```python
from build123d import *

# Parameters (mm, degrees)
F0_W     = 76.2
F0_H     = 177.8
F1_DEPTH = 12.7
F3_D     = 7.62
F4_D     = 7.62
F6_W     = 53.435474
F6_H     = 112.436191
F6_R     = 15.902152
F7_DEPTH = 36.66461


with BuildPart() as f1:
    # F0 (on Top) → F1 (new body)
    with BuildSketch(Plane.XY):
        with Locations((-11.308188, 0.622381)):
            Rectangle(F0_W, F0_H)
    extrude(amount=F1_DEPTH)

    # F3 (through all)
    with Locations(Plane.YZ.offset(26.791812)):
        with Locations((-79.060733, 6.35)):
            Hole(F3_D / 2)

    # F4 (through all)
    with Locations(Plane.YZ.offset(26.791812)):
        with Locations((80.305494, 6.35)):
            Hole(F4_D / 2)

    # F6 (on face) → F7 (join)
    with BuildSketch(Plane.XY.offset(12.7)):
        with Locations((-13.522789, 21.443374)):
            Rectangle(F6_W, F6_H)
        with Locations((-13.522789, 21.443374)):
            Circle(F6_R, mode=Mode.SUBTRACT)
    extrude(amount=F7_DEPTH)


solid = f1.part
```
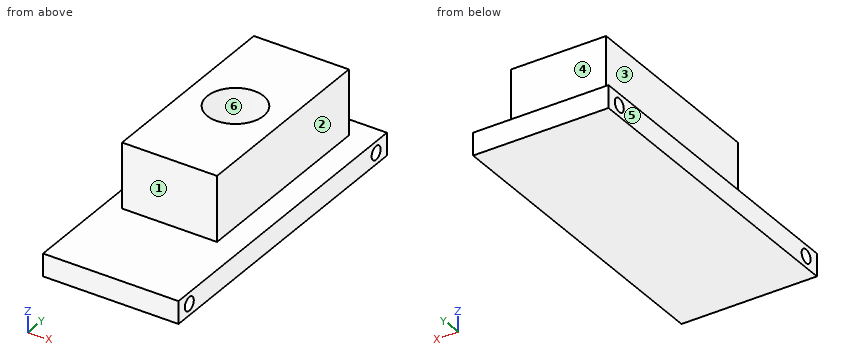
Work out the finished part from the listing and answer in its coordinate system (mm). Face numbers are marked on the shaded views. A direction names the side the tool comes from. Give positions to 0.01 mm unless a question says otherwise; leave off trailing zeros. Loops run counter-clockwise (first coordinate to the right, second up) from the corner with the lowest first, then second, coordinate; pieces in that order, holes last. Notation, with made-up numbers: (17.5, 45) -> (56.5, 45) arc R25 cw to (56.5, 78) -> close; hole circle Ø10 at (-26.5, 36). An arc over 180 degrees is marked (long way). Put each result on its own line as item: value. Start each with the question number.
Item 1: Find the intervals of material crossed by L1, parallel to Y at x = -17, z = 6; L2, parallel to Y at x = -42, z = 3; L3, parallel to Z at x = -29, y = -65, in increasing order. Write a range as [from, to].
Item 2: The mould has two halves that part along Y. Classify the marked faces 4, 5 and 6: released by +Y, released by -Y, zero draft, split by the parting line, or undercut.
Item 3: The part is cut by section B-B (x = -38). Give the vertices of the cut face in (y, z), then the cut area to 3 significant figures.
Item 4: The part is cut by section A-A (z = 6.35). Give the vertices of the cut face in (x, y).
Item 5: The part is cut by section D-D (x = 21.5). Give the vertices of the cut face in (y, z), then the cut area to 3 significant figures.
Item 6: Which of the six approach directions +Z, -Z, +X, -X, +Y, -Y give full straight-line access (tool end or side, diameter ignored) to the marked faces 1, 2 and 3?
Item 7: Each of these flat-tipped pins is pushed along its axis until it touches: P1, Ø16, axis at x = -12.5, y = 23.5, coming from the +Z side; P2, Ø11, axis at y = 26, z = 25, coming from the -X side; P3, Ø6, axis at x = -23, z = 29, coming from the -Y side. Where does it stop, or does it pass through?
Item 8: The part is cut by section C-C (y = -26.5). Give the vertices of the cut face in (x, z).
Answers below:
1. L1: [-88.28, -82.85], [-75.27, 76.51], [84.1, 89.52]
1. L2: [-88.28, -80.88], [-77.25, 78.49], [82.12, 89.52]
1. L3: [0, 12.7]
2. face 4: released by +Y
2. face 5: zero draft
2. face 6: undercut
3. outline: (-88.28, 0) -> (89.52, 0) -> (89.52, 12.7) -> (77.66, 12.7) -> (77.66, 49.36) -> (-34.77, 49.36) -> (-34.77, 12.7) -> (-88.28, 12.7) -> close; hole circle Ø7.62 at (-79.06, 6.35); hole circle Ø7.62 at (80.31, 6.35)
3. area: 6,290 mm2
4. outline: (-49.41, -88.28) -> (26.79, -88.28) -> (26.79, -82.87) -> (-49.41, -82.87) -> close; (-49.41, -75.25) -> (26.79, -75.25) -> (26.79, 76.5) -> (-49.41, 76.5) -> close; (-49.41, 84.12) -> (26.79, 84.12) -> (26.79, 89.52) -> (-49.41, 89.52) -> close
5. outline: (-88.28, 0) -> (89.52, 0) -> (89.52, 12.7) -> (-88.28, 12.7) -> close; hole circle Ø7.62 at (-79.06, 6.35); hole circle Ø7.62 at (80.31, 6.35)
5. area: 2,170 mm2
6. face 1: +Z, +X, -X, -Y
6. face 2: +Z, +X, +Y, -Y
6. face 3: +Z, -X, +Y, -Y
7. P1: z = 12.7
7. P2: x = -40.24
7. P3: y = -34.77
8. outline: (-49.41, 0) -> (26.79, 0) -> (26.79, 12.7) -> (13.19, 12.7) -> (13.19, 49.36) -> (-40.24, 49.36) -> (-40.24, 12.7) -> (-49.41, 12.7) -> close
